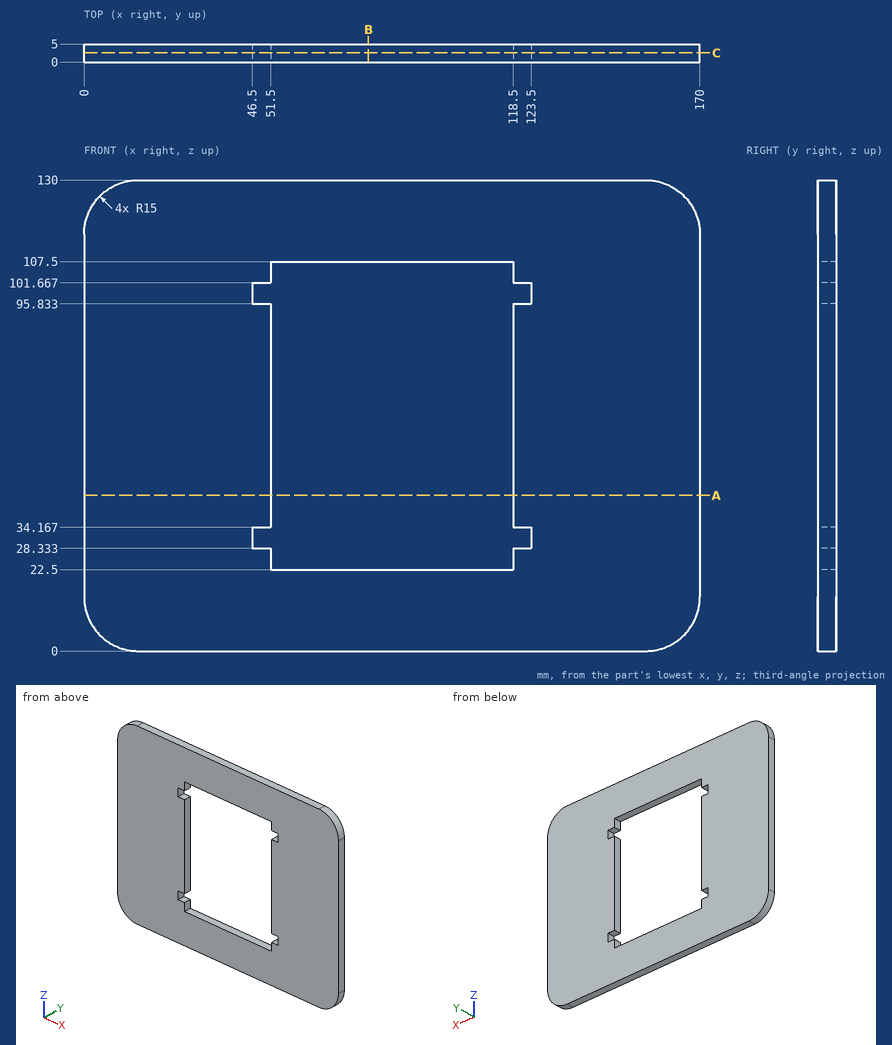
Check sheet for the drawn part. Datum: minimum x, y, z corner. Units: mm. Coordinates: 2 decimals unless noted, no trailing zeros. Order: outer loops, then holes, each group sorted by start corner. A loop starts at its lowest first (then second) coordinate and runs counter-clockwise, first axis right, second up. Notation, with made-up numbers: (82.5, 41.25) -> (131.5, 41.25) arc R22 cw to (131.5, 68.25) -> close; hole circle Ø11 at (10.5, 64). An arc over 180 degrees is marked (long way). Write each question's results on one line, items separated by ' | '. Start each with the question number.
1) Material ranges on line 1 along Z through (x, y) = (50.5, 2.1); line 2 along X through (y, z) = (3.1, 98); line 3 along X through (y, z) = (2.95, 24), recorded low to high.
2) Depth check by flat-ended pin: pin 1 (2.5 mm diameter, centred on y = 2.5, z = 104.5, fed in from -X). Enter the tip coordinate at first touch or a pass-through.
3) Section check A-A (z = 43). Enter the section's corners in (x, y).
4) Section check B-B (x = 78.5). Enter the section's corners in (y, z).
5) Section check C-C (y = 2.55). Enter the section's corners in (x, z).
Checked values:
1) line 1: 0 to 28.33, 34.17 to 95.83, 101.67 to 130 | line 2: 0 to 46.5, 123.5 to 170 | line 3: 0 to 51.5, 118.5 to 170
2) pin 1: x = 0
3) outline: (0, 0) -> (51.5, 0) -> (51.5, 5) -> (0, 5) -> close; (118.5, 0) -> (170, 0) -> (170, 5) -> (118.5, 5) -> close
4) outline: (0, 0) -> (5, 0) -> (5, 22.5) -> (0, 22.5) -> close; (0, 107.5) -> (5, 107.5) -> (5, 130) -> (0, 130) -> close
5) outline: (0, 15) arc R15 ccw to (15, 0) -> (155, 0) arc R15 ccw to (170, 15) -> (170, 115) arc R15 ccw to (155, 130) -> (15, 130) arc R15 ccw to (0, 115) -> close; hole (46.5, 28.33) -> (51.5, 28.33) -> (51.5, 22.5) -> (118.5, 22.5) -> (118.5, 28.33) -> (123.5, 28.33) -> (123.5, 34.17) -> (118.5, 34.17) -> (118.5, 95.83) -> (123.5, 95.83) -> (123.5, 101.67) -> (118.5, 101.67) -> (118.5, 107.5) -> (51.5, 107.5) -> (51.5, 101.67) -> (46.5, 101.67) -> (46.5, 95.83) -> (51.5, 95.83) -> (51.5, 34.17) -> (46.5, 34.17) -> close
